```python
from build123d import *

# Parameters (mm, degrees)
F0_W     = 38.1
F0_H     = 12.7
F1_DEPTH = 12.7
F3_DEPTH = 25.4
F4_W     = 38.1
F4_H     = 12.7
F5_DEPTH = 12.7


with BuildPart() as f1:
    # F0 (on Front) → F1 (new body)
    with BuildSketch(Plane.XZ):
        with Locations((-19.05, 6.35)):
            Rectangle(F0_W, F0_H)
    extrude(amount=F1_DEPTH)

    # F2 (on face) → F3 (cut)
    with BuildSketch(Plane.XY.offset(12.7)):
        Polygon((0, -12.7), (0, 0), (-12.7, -12.7), align=None)
    extrude(amount=-F3_DEPTH, mode=Mode.SUBTRACT)

    # F4 (on face) → F5 (join)
    with BuildSketch(Plane(origin=(0, 0, 0), x_dir=(-1, 0, 0), z_dir=(0, 1, 0))):
        with Locations((19.05, 6.35)):
            Rectangle(F4_W, F4_H)
        Polygon((0, 12.7), (38.1, 12.7), (38.1, 34.697045), (12.7, 34.697045), align=None)
    extrude(amount=F5_DEPTH)


solid = f1.part
```
Here's how the part is built. I have some questions about the finished solid (model axes, mm). A direction names the side the tool comes from. Round coordinates to 2 decimals unless told otherwise and drop trailing zeros. Order: outer loops, then holes, each group sorted by start corner. A loop starts at its lowest first (then second) coordinate and runs counter-clockwise, first axis right, second up. Notation, with made-up numbers: M 78,-17.75 L 102,-17.75 A31 ccw 102,6.25 Z; hole C 70,24.25 d10. An arc over 180 degrees is marked long. Answer as CSV lines item,"result".
Item 1: For pin 1 (8 mm diameter, centred on x = -19.5, z = 26, fed in from -Y); pin 2 (4 mm diameter, centred on x = -25, y = -4, fed in from +Z); pin 3 (4 mm diameter, centred on x = -19, y = -2.5, fed in from -Z); pin 4 (5 mm diameter, centred on y = 2, z = 30, fed in from +X), each with a flat end and sliding along its axis, tell me the tip position at first contact or that it passes through.
From the geometry:
pin 1,"y = 0"
pin 2,"z = 12.7"
pin 3,"z = 0"
pin 4,"x = -8.54"
Item 2: Imagine slicing it at B-B on y = 2.75. List the corners of the cut face in (x, z) for me, and give its area (3 significant figures).
From the geometry:
outline,"M -38.1,0 L 0,0 L 0,12.7 L -12.7,34.7 L -38.1,34.7 Z"
area,"1,180 mm2"
Item 3: Imagine slicing it at C-C on x = -34. List the corners of the cut face in (y, z) for me.
From the geometry:
outline,"M -12.7,0 L 12.7,0 L 12.7,34.7 L 0,34.7 L 0,12.7 L -12.7,12.7 Z"
Item 4: Which directions (+Z, -Z, +X, -X, +Y, -Y) give clear straight access to the entire face, cutting with the end or side of a thin tool? Please do faces 1 (the flat face through (-24, -6, 12.7)), 2 (the flat face through (-26, -12.7, 6)).
From the geometry:
face 1,"+Z, +X, -X, -Y"
face 2,"+Z, -Z, +X, -X, -Y"
Item 5: Imagine slicing it at A-A on z = 11. List the corners of the cut face in (x, y) for me.
From the geometry:
outline,"M -38.1,-12.7 L -12.7,-12.7 L 0,0 L 0,12.7 L -38.1,12.7 Z"
Item 6: Imagine slicing it at D-D on x = -6. List the corners of the cut face in (y, z) for me.
From the geometry:
outline,"M -6,0 L 12.7,0 L 12.7,23.09 L 0,23.09 L 0,12.7 L -6,12.7 Z"
Item 7: Please list where these lines run through material, in increasing order: L1, parallel to Y at x = -21.5, z = 26.5; L2, parallel to Z at x = -4.5, y = 4.25. Write a range as [from, to].
From the geometry:
L1,"[0, 12.7]"
L2,"[0, 20.49]"
